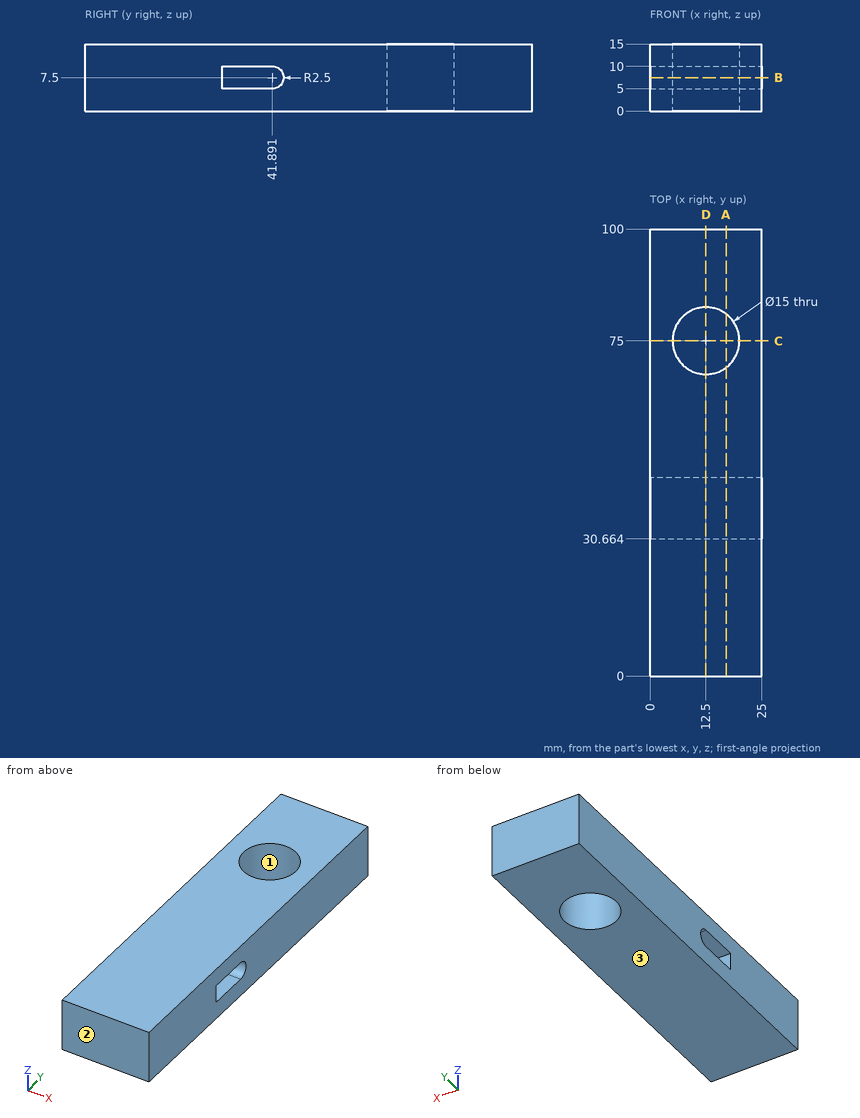
Answer from the drawing. Dimensions are ordinates in mm from the lowest x, y and z of the part. Give positions to 0.01 mm unless a question says otherwise; leave off trailing zeros. Loops run counter-clockwise (first coordinate to the right, second up) from the corner with the lowest first, then second, coordinate; pieces in that order, holes last. Notation, with made-up numbers: (-26, 12.25) - (-19, 12.25) arc R18 ccw to (-19, 43.25) - close; hole circle Ø1 at (-19, -20.5). An arc over 180 degrees is marked (long way). Write each question's results on one line, items separated by ' | '.
1. Find section B-B, the plane z = 7.5. Write down the section's boundary in (x, y).
Resolved:
outline: (0, 0) - (25, 0) - (25, 30.66) - (0, 30.66) - close; (0, 44.39) - (25, 44.39) - (25, 100) - (0, 100) - close; hole circle Ø15 at (12.5, 75)
2. Find section D-D, the plane x = 12.5. Write down the section's boundary in (y, z).
Resolved:
outline: (0, 0) - (67.5, 0) - (67.5, 15) - (0, 15) - close; (82.5, 0) - (100, 0) - (100, 15) - (82.5, 15) - close; hole (30.66, 5) - (41.89, 5) arc R2.5 ccw to (41.89, 10) - (30.66, 10) - close
3. Find section C-C, the plane y = 75. Write down the section's boundary in (x, z).
Resolved:
outline: (0, 0) - (5, 0) - (5, 15) - (0, 15) - close; (20, 0) - (25, 0) - (25, 15) - (20, 15) - close
4. A flat-ended cylindrical pin translates along its axis: P1, Ø12, axis at x = 12.5, y = 75, coming from the +Z side. Find the tip coordinate at first contact, or state that the pin passes through.
Resolved:
P1: passes through
5. For a pull along Y with two mould halves and no side action, classify the marked faces 1, 2 and 3 as +Y half, -Y half, draft (parallel to the pull), parting line (faces both ways), or undercut.
Resolved:
face 1: undercut | face 2: -Y half | face 3: draft
6. Find section A-A, the plane x = 17. Write down the section's boundary in (y, z).
Resolved:
outline: (0, 0) - (69, 0) - (69, 15) - (0, 15) - close; (81, 0) - (100, 0) - (100, 15) - (81, 15) - close; hole (30.66, 5) - (41.89, 5) arc R2.5 ccw to (41.89, 10) - (30.66, 10) - close
7. Consider probe 1 along Y at (x, z) = (12.5, 10.25); probe 2 along Y at (x, z) = (12.5, 7.25); probe 3 along Z at (x, y) = (11, 34.5). Determine where each line is inside the solid, lowest interval first. Write a range as from..to.
Resolved:
probe 1: y = 0..67.5, 82.5..100 | probe 2: y = 0..30.66, 44.38..67.5, 82.5..100 | probe 3: z = 0..5, 10..15
